Build history of the part. All positions in model axes, mm. A direction names the side the tool comes from. Give positions to 0.01 mm unless a question says otherwise; leave off trailing zeros. Loops run counter-clockwise (first coordinate to the right, second up) from the corner with the lowest first, then second, coordinate; pieces in that order, holes last. Notation, with made-up numbers: (76, 52) -> (129, 52) arc R27 ccw to (129, 88) -> close; hole circle Ø4 at (-20.75, 32). An arc over 180 degrees is marked (long way). Answer as a JSON object with one key per item and string values. Group by question number.
from build123d import *

# Parameters (mm, degrees)
SKETCH_R   = 8
SKETCH_R_2 = 3
PAD_DEPTH  = 10


with BuildPart() as part:
    # Sketch → Pad (new body)
    with BuildSketch(Plane.XY):
        Polygon((-25, 45), (55, 45), (55, -75), (40, -75), (40, -62.235413), (7.625615, -16), (-25, -16), align=None)
        Circle(SKETCH_R, mode=Mode.SUBTRACT)
        with Locations((40, -52)):
            Circle(SKETCH_R_2, mode=Mode.SUBTRACT)
        with Locations((40, 22)):
            Circle(SKETCH_R_2, mode=Mode.SUBTRACT)
        with Locations((-10, 22)):
            Circle(SKETCH_R_2, mode=Mode.SUBTRACT)
    extrude(amount=PAD_DEPTH)


solid = part.part
(1) Saw through at A-A on y = 0. List the corners of the cut face in (x, z).
(2) Saw through at D-D on y = 22. List the corners of the cut face in (x, z), plus the area to 3 significant figures.
(3) Saw through at C-C on x = -10. List the corners of the cut face in (y, z), plus the area to 3 significant figures.
(4) 3-axis set-ups, long thin cutter, end or side, ignore diameter. For faces 4 (the flat face through (-8, -16, 5)), 5 (the flat face through (14, 45, 5)): which of +Z, -Z, +X, -X, +Y, -Y reach the whole face in a straight line?
(5) Saw through at B-B on z = 6.25. List the corners of the cut face in (x, y).
(6) Probe line 1 along Y through (x, z) = (-10, 6.75); line 2 along Y through (x, z) = (0, 5.5); line 3 along Y through (x, z) = (-18, 1.75). List the from-to ranges inside material, lowest first. Write a range as [from, to].
(7) Pull direction Y, two halves, no side cores. Call faces 1 (the cylindrical face through (37, 22, 5)), 2 (the flat face through (-25, 14, 5)), 3 (the flat face through (48, -75, 5)): pulls with the +Y half, pulls with the -Y half, needs draft (parallel to the pull), parting line crosses it, or undercut.
(8) Pin check, flat tips, straight feed: pin 1 (3 mm diameter, centred on x = -10, z = 7, fed in from -Y); pin 2 (5 mm diameter, centred on x = 23, z = 4.5, fed in from -Y); pin 3 (6 mm diameter, centred on y = -21.5, z = 5.5, fed in from -X). Stop position of each tip, or through.
Calculated:
{
 "1": {"outline": "(-25, 0) -> (-8, 0) -> (-8, 10) -> (-25, 10) -> close; (8, 0) -> (55, 0) -> (55, 10) -> (8, 10) -> close"},
 "2": {"outline": "(-25, 0) -> (-13, 0) -> (-13, 10) -> (-25, 10) -> close; (-7, 0) -> (37, 0) -> (37, 10) -> (-7, 10) -> close; (43, 0) -> (55, 0) -> (55, 10) -> (43, 10) -> close", "area": "680 mm^2"},
 "3": {"outline": "(-16, 0) -> (19, 0) -> (19, 10) -> (-16, 10) -> close; (25, 0) -> (45, 0) -> (45, 10) -> (25, 10) -> close", "area": "550 mm^2"},
 "4": {"face 4": "+Z, -Z, -X, -Y", "face 5": "+Z, -Z, +X, -X, +Y"},
 "5": {"outline": "(-25, -16) -> (7.63, -16) -> (40, -62.24) -> (40, -75) -> (55, -75) -> (55, 45) -> (-25, 45) -> close; hole circle Ø6 at (-10, 22); hole circle Ø16 at (0, 0); hole circle Ø6 at (40, -52); hole circle Ø6 at (40, 22)"},
 "6": {"line 1": "y = [-16, 19], [25, 45]", "line 2": "y = [-16, -8], [8, 45]", "line 3": "y = [-16, 45]"},
 "7": {"face 1": "undercut", "face 2": "needs draft", "face 3": "pulls with the -Y half"},
 "8": {"pin 1": "stops at y = -16", "pin 2": "stops at y = -41.53", "pin 3": "stops at x = 9.38"}
}
